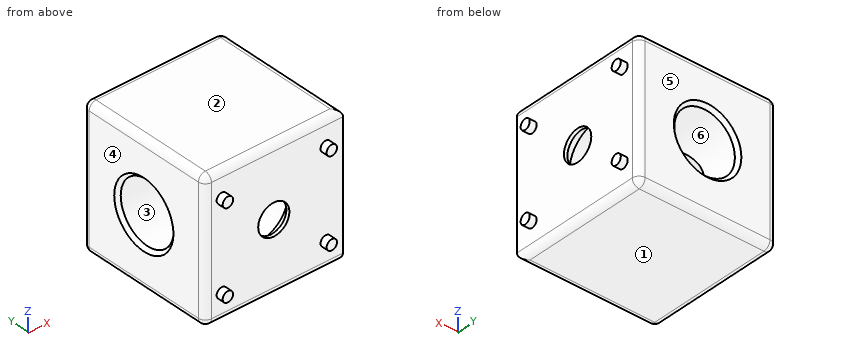
```python
from build123d import *

# Parameters (mm, degrees)
SKETCH_1_W      = 40
SKETCH_1_H      = 40
EXTRUDE_1_DEPTH = 20
SKETCH_5_R      = 1.5
EXTRUDE_2_DEPTH = 2
FILLET_1_R      = 2


with BuildPart() as part:
    # Эскиз1 → Бобышка-Вытянуть1 (new body, symmetric)
    with BuildSketch(Plane(origin=(0, 0, 0), x_dir=(1, 0, 0), z_dir=(0, 1, 0))):
        Rectangle(SKETCH_1_W, SKETCH_1_H)
    extrude(amount=EXTRUDE_1_DEPTH, both=True)

    # Эскиз4 → Вырез-Повернуть1 (revolve, cut)
    with BuildSketch(Plane.XY):
        Polygon((-4.5, -20), (-4.5, -19), (-8.75, -14.75), (-8.75, 19), (-9.75, 20), (0, 20), (0, -20), align=None)
    cut_revolve_1 = revolve(axis=Axis((0, 20, 0), (0, -1, 0)), mode=Mode.SUBTRACT)

    # Эскиз5 → Бобышка-Вытянуть2 (add)
    with BuildSketch(Plane.XZ.offset(20)):
        with Locations(Location((-15, 12.5, 0), (0, 0, 270))):  # turned: the seam where the file's is
            Circle(SKETCH_5_R)
        with Locations(Location((-15, -12.5, 0), (0, 0, 270))):  # turned: the seam where the file's is
            Circle(SKETCH_5_R)
        with Locations(Location((15, -12.5, 0), (0, 0, 270))):  # turned: the seam where the file's is
            Circle(SKETCH_5_R)
        with Locations(Location((15, 12.5, 0), (0, 0, 270))):  # turned: the seam where the file's is
            Circle(SKETCH_5_R)
    extrude_2 = extrude(amount=EXTRUDE_2_DEPTH)

    # Зеркальное отражение1: Вырез-Повернуть1, Бобышка-Вытянуть2 across plane
    add(cut_revolve_1.mirror(Plane(origin=(0, 0, 0), x_dir=(0, 0, 1), z_dir=(0.707106781, 0.707106781, 0))), mode=Mode.SUBTRACT)
    add(extrude_2.mirror(Plane(origin=(0, 0, 0), x_dir=(0, 0, 1), z_dir=(0.707106781, 0.707106781, 0))))

    # Скругление1
    fillet_1_edges = [part.edges().sort_by_distance(p)[0] for p in [
        (-20, 20, 0),
        (0, 20, 20),
        (20, 20, 0),
        (0, -20, 20),
        (-20, -20, 0),
        (0, -20, -20),
        (20, 0, 20),
        (-20, 0, 20),
        (-20, 0, -20),
        (20, 0, -20),
        (0, 20, -20),
    ]]
    fillet(fillet_1_edges, radius=FILLET_1_R)


solid = part.part
```
Here's how the part is built. I have some questions about the finished solid (model axes, mm). Face numbers are marked on the shaded views. A direction names the side the tool comes from. Give positions to 0.01 mm unless a question says otherwise; leave off trailing zeros. Loops run counter-clockwise (first coordinate to the right, second up) from the corner with the lowest first, then second, coordinate; pieces in that order, holes last. Notation, with made-up numbers: M 19,63.5 L 32,63.5 A31 ccw 32,96.5 Z; hole C -6,8 d5. An arc over 180 degrees is marked long. Use one line per item in the form item = value. Start each with the question number.
Q1. Will these pins go through, and if not, where does the flat tip stop? pin 1 Ø2 at (x, z) = (-12, 5) entering from -Y; pin 2 Ø18 at (y, z) = (1, 5) entering from +X; pin 3 Ø8 at (x, z) = (10.5, 12.5) entering from -Y; pin 4 Ø10.5 at (y, z) = (0, 0) entering from -X.
Q2. I need wall thicknesses on line 1 along Y through (x, z) = (-16.5, 0.5); line 2 along Z through (x, y) = (4.25, 0); line 3 along Y through (x, z) = (16, -6). Which ranges of each line are inside material? Lowest first, please.
Q3. Thinking about a two-plate mould opening in Z: for the marked faces 1, 2, 3 and 4, which applies, +Z half, -Z half, draft (parallel to the pull), parting line (faces both ways), or undercut?
Q4. Which directions (+Z, -Z, +X, -X, +Y, -Y) give clear straight access to the entire face, cutting with the end or side of a thin tool? Please do the marked faces 5 and 6.
Q5. If we section it at A-A (y = 12.5): Write out the boundary of the cut face in (x, z).
Q6. If we section it at D-D (z = -12.5): Write out the boundary of the cut face in (x, y), then the cut area to 3 significant figures.
Q7. If we section it at C-C (z = -17): Write out the boundary of the cut face in (x, y).
Taken from the geometry:
q1.pin_1 = -20
q1.pin_2 = 20
q1.pin_3 = -22
q1.pin_4 = 18.25
q2.line_1 = -20 to -8.74, 8.74 to 20
q2.line_2 = -20 to -8.75, 8.75 to 20
q2.line_3 = -20 to -4.5, 4.5 to 20
q3.face_1 = -Z half
q3.face_2 = +Z half
q3.face_3 = undercut
q3.face_4 = draft
q4.face_5 = +Z, -Z, +X, -X, +Y
q4.face_6 = +Y
q5.outline = M -20,-18 A2 ccw -18,-20 L 18,-20 A2 ccw 20,-18 L 20,18 A2 ccw 18,20 L -18,20 A2 ccw -20,18 Z; hole C 0,0 d17.5
q6.outline = M -20,-18 A2 ccw -18,-20 L -16.5,-20 L -16.5,-22 L -13.5,-22 L -13.5,-20 L 13.5,-20 L 13.5,-22 L 16.5,-22 L 16.5,-20 L 20,-20 L 20,-16.5 L 22,-16.5 L 22,-13.5 L 20,-13.5 L 20,13.5 L 22,13.5 L 22,16.5 L 20,16.5 L 20,18 A2 ccw 18,20 L -18,20 A2 ccw -20,18 Z
q6.area = 1,620 mm^2
q7.outline = M -20,-18 A2 ccw -18,-20 L 20,-20 L 20,18 A2 ccw 18,20 L -18,20 A2 ccw -20,18 Z
